Model file for the job. Use its own axes, mm. A direction names the side the tool comes from. Coordinates: 2 decimals unless noted, no trailing zeros. Write each loop counter-clockwise with the first axis right and the second up, starting at its lowest first coordinate (ties: lowest second). Pieces come first, ordered by that corner, then holes. Notation, with made-up numbers: M 29.25,49 L 43.25,49 A29 cw 43.25,76 Z; hole C 4.5,63.5 d4. An arc over 180 degrees is marked long. Put each result on its own line as item: value. Start each with the question number.
Q1. Drill centre lines: line 1 along X through (y, z) = (17.5, -10); line 2 along X through (y, z) = (11.75, -85); line 3 along X through (y, z) = (6.25, -78.25). Where is each one in solid material? Low to high.
Q2. Cut at B-B (x = -46). Write the cut outline in (y, z), then the cut area to 3 significant figures.
Q3. Which spindle directions (+Z, -Z, +X, -X, +Y, -Y) get a long thin tool onto all of the face, cutting with end or side? Do faces 1 (the flat face through (-35.024, 15, 50)), 2 (the flat face through (-70, 15, -80)), 3 (the flat face through (67, 15, 80.062)). Say none if no direction does.
Q4. Pull direction Z, two halves, no side cores. Call faces 4 (the flat face through (-100, 10, -1)), 5 (the flat face through (0, 15, 20.062)), 6 (the flat face through (-16, 5, 0)), 7 (the flat face through (0, 5, -16)): pulls with the +Z half, pulls with the -Z half, needs draft (parallel to the pull), parting line crosses it, or undercut.
Q5. Drop flat-ended pins along their axis: pin 1 (4 mm diameter, centred on x = 10, z = 10, fed in from +Y); pin 2 (8 mm diameter, centred on x = -16, y = 15.5, fed in from +Z). Give the stop position or say it passes through.
Q6. Cut at A-A (y = 15.75). Give the number of separate pieces and of enclosed holes in the cut face, then the cut area to 3 significant figures.
Autodesk Inventor part; units mm, degrees
ref_plane "YZ Plane" through (0, 0, 0) normal (1, 0, 0) x (0, 1, 0)
ref_plane "XZ Plane" through (0, 0, 0) normal (0, 1, 0) x (-1, 0, 0)
ref_plane "XY Plane" through (0, 0, 0) normal (0, 0, 1) x (1, 0, 0)
sketch "Boceto1" plane through (0, 0, 0) normal (0, 1, 0) x (-1, 0, 0)
  line L0 (100, 100) -> (-100, 100)
  line L1 (-100, 100) -> (-100, -100)
  line L2 (-100, -100) -> (100, -100)
  line L3 (100, -100) -> (100, 100)
  line L4 (100, 100) -> (-100, -100) construction
  line L5 (-100, 100) -> (100, -100) construction
  point P0 (0, 0)
  dimension "d0" = 200
  dimension "d1" = 200
extrude "Extrusión1" add sketch "Boceto1" along normal blind 20
sketch "Boceto2" plane through (0, 20, 0) normal (0, 1, 0) x (1, 0, 0)
  circle A0 centre (-11.5239, -30.0616) radius 3
  circle A1 centre (11.4761, -30.0616) radius 3
  circle A2 centre (-11.5239, -60.0616) radius 3
  circle A3 centre (11.4761, -60.0616) radius 3
  line L0 (-0.0239, -45.0616) -> (-35.0239, -45.0616)
  line L1 (-35.0239, -45.0616) -> (-35.0239, -80.0616)
  line L2 (-0.0239, -45.0616) -> (34.9761, -45.0616)
  line L3 (-11.5239, -30.0616) -> (11.4761, -60.0616)
  line L4 (-11.5239, -60.0616) -> (11.4761, -30.0616)
  line L5 (34.9761, -20.0616) -> (-35.0239, -20.0616)
  line L6 (-35.0239, -20.0616) -> (-35.0239, -80.0616)
  line L7 (34.9761, -80.0616) -> (34.9761, -20.0616)
  line L8 (-105, -100.0616) -> (105, -100.0616)
  line L9 (-105.0239, -80.0616) -> (104.9761, -80.0616)
  line L10 (-35.0239, -80.0616) -> (34.9761, -80.0616)
  line L11 (105, -100.0616) -> (95.8154, -100.0616)
  line L12 (-105.0239, -80.0616) -> (104.9761, -80.0616)
  line L13 (105, -80.0616) -> (-105, -80.0616)
  line L14 (-105, -100.0616) -> (105, -100.0616)
  line L15 (105, -90.0616) -> (94.0798, -90.0616)
  line L16 (-105, -100.0616) -> (105, -100.0616)
  line L17 (-105, -80.0616) -> (105, -80.0616)
  line L18 (105, -80.0616) -> (105, -100.0616)
  line L19 (105, -100.0616) -> (-105, -100.0616)
  line L20 (-105, -100.0616) -> (-105, -80.0616)
  line L21 (-100, 100) -> (-100, -100)
  line L22 (-100, -100) -> (100.4077, -100)
  point P0 (0, 0)
  point P1 (0, -10.0616)
  point P2 (0, -90.0616)
  point P3 (-0.0478, -80.0616)
  dimension "d4" = 20
  dimension "d5" = 20
  dimension "d6" = 30
  dimension "d7" = 30
  dimension "d8" = 20
  dimension "d9" = 35
  dimension "d10" = 35
  dimension "d11" = 60
extrude "Extrusión2" cut sketch "Boceto2" against normal blind 10
sketch "Boceto3" plane through (0, 20, 0) normal (0, 1, 0) x (1, 0, 0)
  circle A0 centre (-11.5239, -30.0616) radius 3
  circle A1 centre (-11.5239, -30.0616) radius 3
  circle A2 centre (11.4761, -30.0616) radius 3
  circle A3 centre (11.4761, -30.0616) radius 3
  circle A4 centre (11.4761, -60.0616) radius 3
  circle A5 centre (11.4761, -60.0616) radius 3
  circle A6 centre (-11.5239, -60.0616) radius 3
  point P0 (0, 0)
extrude "Extrusión3" cut sketch "Boceto3" against normal blind 20
sketch "Boceto4" plane through (0, 20, 0) normal (0, 1, 0) x (1, 0, 0)
  circle A0 centre (-51.75, 78.25) radius 1.75
  line L0 (-50, 70) -> (-60, 70)
  line L1 (-60, 70) -> (-60, 80)
  line L2 (-60, 80) -> (-50, 80)
  line L3 (-50, 80) -> (-50, 70)
  line L4 (-50, 70) -> (-60, 80) construction
  line L5 (-60, 70) -> (-50, 80) construction
  line L6 (-105, 90) -> (-105, -90)
  circle A1 centre (-58.25, 71.75) radius 1.75
  line L7 (0, 90) -> (0, 77.3124)
  circle A2 centre (51.75, 78.25) radius 1.75
  line L8 (50, 70) -> (60, 70)
  line L9 (60, 70) -> (60, 80)
  line L10 (60, 80) -> (50, 80)
  line L11 (50, 80) -> (50, 70)
  line L12 (50, 70) -> (60, 80) construction
  line L13 (60, 70) -> (50, 80) construction
  circle A3 centre (58.25, 71.75) radius 1.75
  line L14 (100, 100) -> (-100, 100)
  line L15 (-100, 100) -> (-100, -80.0616)
  line L16 (100, -80.0616) -> (100, 100)
  point P0 (0, 0)
  point P1 (0, 0)
  point P2 (-60, 75)
  point P3 (60, 75)
  dimension "d16" = 3.5
  dimension "d18" = 1.75
  dimension "d19" = 1.75
  dimension "d20" = 1.75
  dimension "d21" = 1.75
  dimension "d22" = 10
  dimension "d23" = 10
  dimension "d25" = 20
  dimension "d26" = 40
  dimension "d27" = 40
hole "Agujero1" at (-58.25, 20, -71.75) at (-51.75, 20, -78.25) at (58.25, 20, -71.75) at (51.75, 20, -78.25) direction (0, -1, 0) diameter 3.5 end through all
sketch "Boceto5" plane through (0, 20, 0) normal (0, 1, 0) x (1, 0, 0)
  line L0 (0, 90) -> (0, 68.25)
  circle A0 centre (-51.75, 78.25) radius 1.75
  line L1 (-50, 78.25) -> (-50, 100)
  circle A1 centre (-58.25, 71.75) radius 1.75
  line L2 (-60, 71.75) -> (-60, 100)
  line L3 (-60, 100) -> (-70, 100)
  line L4 (-50, 100) -> (-40, 100)
  line L5 (-40, 100) -> (-40, 60)
  line L6 (-40, 60) -> (-70, 60)
  line L7 (-70, 60) -> (-70, 100)
  line L8 (-70, 100) -> (-40, 100)
  circle A2 centre (51.75, 78.25) radius 1.75
  line L9 (50, 78.25) -> (50, 100)
  circle A3 centre (58.25, 71.75) radius 1.75
  line L10 (60, 71.75) -> (60, 100)
  line L11 (60, 100) -> (70, 100)
  line L12 (50, 100) -> (40, 100)
  line L13 (40, 100) -> (40, 60)
  line L14 (40, 60) -> (70, 60)
  line L15 (70, 60) -> (70, 100)
  line L16 (70, 100) -> (40, 100)
  point P0 (0, 0)
  dimension "d38" = 10
  dimension "d39" = 10
  dimension "d40" = 40
extrude "Extrusión4" cut sketch "Boceto5" against normal blind 10
ref_plane "Plano de trabajo1" through (0, 0, -100) normal (-1, 0, 0) x (0, 0, 1)
ref_plane "Plano de trabajo2" through (100, 0, 0) normal (0, 0, -1) x (-1, 0, 0)
sketch "Boceto7" plane through (0, 0, 0) normal (0, -1, 0) x (1, 0, 0)
  circle A0 centre (10, -10) radius 1.75
  line L0 (6.803, 0) -> (14.6069, 0)
  line L1 (0, 0) -> (0, -4.8284)
  line L2 (0, 0) -> (20.0354, 0)
  circle A1 centre (10, 10) radius 1.75
  line L3 (0, 0) -> (0, 4.8284)
  circle A2 centre (-10, -10) radius 1.75
  circle A3 centre (-10, 10) radius 1.75
  dimension "d52" = 3.5
  dimension "d54" = 10
  dimension "d55" = 10
hole "Agujero2" at (10, 0, -10) at (10, 0, 10) at (-10, 0, 10) at (-10, 0, -10) direction (0, 1, 0) diameter 3.5 end through all
sketch "Boceto8" plane through (0, 0, 0) normal (0, -1, 0) x (1, 0, 0)
  line L0 (-16, 16) -> (16, 16)
  line L1 (16, 16) -> (16, -16)
  line L2 (16, -16) -> (-16, -16)
  line L3 (-16, -16) -> (-16, 16)
  line L4 (-16, 16) -> (16, -16) construction
  line L5 (16, 16) -> (-16, -16) construction
  point P0 (0, 0)
  dimension "d63" = 32
  dimension "d64" = 32
extrude "Extrusión5" cut sketch "Boceto8" against normal blind 10
sketch "Boceto9" plane through (0, 0, 0) normal (0, -1, 0) x (1, 0, 0)
  circle A0 centre (85, -10) radius 1.75
  line L0 (100, 100) -> (100, -100)
  line L1 (140, 0) -> (-140, 0)
  circle A1 centre (85, 10) radius 1.75
  line L2 (0, 0) -> (0, 9.4908)
  circle A2 centre (-85, -10) radius 1.75
  circle A3 centre (-85, 10) radius 1.75
  line L3 (0, 0) -> (6.3157, 6.3157)
  line L4 (0, 0) -> (8.9318, 0) construction
  circle A4 centre (10, 85) radius 1.75
  circle A5 centre (-10, -85) radius 1.75
  line L5 (0, 0) -> (5.9531, -5.9531)
  line L6 (0, 0) -> (8.419, 0) construction
  circle A6 centre (10, -85) radius 1.75
  circle A7 centre (-10, 85) radius 1.75
  dimension "d67" = 3.5
  dimension "d68" = 15
  dimension "d69" = 10
  dimension "d70" = 45
  dimension "d71" = 45
hole "Agujero3" at (-10, 0, 85) at (10, 0, 85) at (85, 0, 10) at (85, 0, -10) at (-85, 0, 10) at (-85, 0, -10) at (-10, 0, -85) at (10, 0, -85) direction (0, 1, 0) diameter 3.5 end through all
properties part number "base_front_red"
Computed values:
1. line 1: -100 to -86.75, -83.25 to -11.75, -8.25 to 8.25, 11.75 to 83.25, 86.75 to 100
1. line 2: -100 to -70, -40 to -11.75, -8.25 to 8.25, 11.75 to 40, 70 to 100
1. line 3: -100 to -53.5, -50 to 50, 53.5 to 100
2. outline: M 0,-100 L 10,-100 L 10,-60 L 20,-60 L 20,80.06 L 10,80.06 L 10,100 L 0,100 Z
2. area: 3,400 mm2
3. face 1: +Z, +Y
3. face 2: -Z, +Y
3. face 3: +Z, +X, -X, +Y
4. face 4: needs draft
4. face 5: pulls with the +Z half
4. face 6: undercut
4. face 7: undercut
5. pin 1: y = 20
5. pin 2: z = 20.06
6. separate pieces: 1
6. enclosed holes: 10
6. area: 29,300 mm2
